CAD build for the part. Positions are in the model's coordinates, mm. Face numbers are marked on the shaded views. A direction names the side the tool comes from. Give positions to 0.01 mm unless a question says otherwise; leave off trailing zeros. Write each loop counter-clockwise with the first axis right and the second up, starting at its lowest first coordinate (ties: lowest second). Pieces come first, ordered by that corner, then holes. Notation, with made-up numbers: (69, 18) -> (112, 18) arc R20 ccw to (112, 42) -> close; hole circle Ø11 at (-1, 37.25). An arc over 180 degrees is marked (long way). Answer in a Markdown table with one row per item. Add a question column.
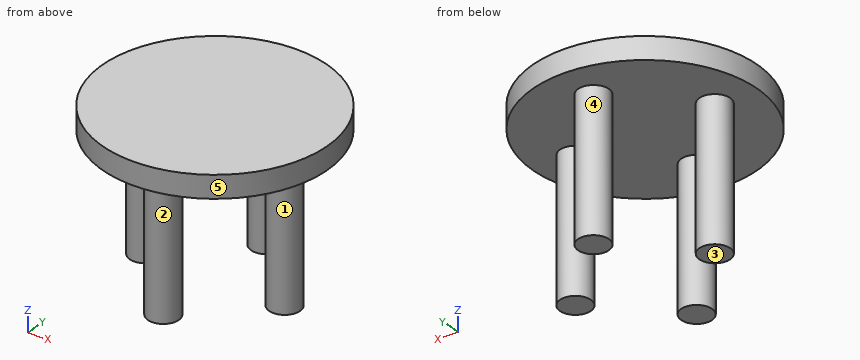
```python
from build123d import *

# Parameters (mm, degrees)
SKETCH_R     = 40
PAD_DEPTH    = 8
SKETCH001_R  = 5.5
PAD001_DEPTH = 50


with BuildPart() as part:
    # Sketch → Pad (new body)
    with BuildSketch(Plane.XY):
        Circle(SKETCH_R)
    extrude(amount=PAD_DEPTH)

    # Sketch001 → Pad001 (new body)
    with BuildSketch(Plane(origin=(0, 0, 0), x_dir=(1, 0, 0), z_dir=(0, 0, -1))):
        with Locations((0, 25)):
            Circle(SKETCH001_R)
        with Locations((-25, 0)):
            Circle(SKETCH001_R)
        with Locations((0, -25)):
            Circle(SKETCH001_R)
        with Locations((25, 0)):
            Circle(SKETCH001_R)
    extrude(amount=PAD001_DEPTH)


solid = part.part
```
Item 1: Drop flat-ended pins along their axis: pin 1 Ø8 at (y, z) = (22, -19) entering from +X; pin 2 Ø1 at (x, z) = (23, -39.5) entering from +Y; pin 3 Ø12 at (y, z) = (-21.5, -8.5) entering from -X. Give the stop position or say it passes through.
Item 2: Slice it at D-D, the plane y = -32. List the corners of the cut face in (x, z).
Item 3: Which spindle directions (+Z, -Z, +X, -X, +Y, -Y) get a long thin tool onto all of the face, cutting with end or side? Do the marked faces 4 and 5. Say none if no direction does.
Item 4: Probe L1, parallel to Z at x = -17, y = 12.5; L2, parallel to Y at x = -2.5, z = -10; L3, parallel to Y at x = 4.5, z = -3.5. List the from-to ranges inside material, lowest first. Write a range as from..to.
Item 5: Mould opens along X. For the marked faces 1, 2 and 3 say: released by +X, released by -X, zero draft, split by the parting line, or undercut.
Item 6: Slice it at A-A, the plane x = 0. List the corners of the cut face in (y, z).
Item 7: Slice it at B-B, the plane z = -17. List the corners of the cut face in (x, y).
Answer key:
| question | item | result |
|---|---|---|
| 1 | pin 1 | stops at x = 5.5 |
| 1 | pin 2 | stops at y = 5.29 |
| 1 | pin 3 | stops at x = -5.5 |
| 2 | outline | (-24, 0) -> (24, 0) -> (24, 8) -> (-24, 8) -> close |
| 3 | face 4 | -Z |
| 3 | face 5 | +Z, -Z |
| 4 | L1 | z = 0..8 |
| 4 | L2 | y = -29.9..-20.1, 20.1..29.9 |
| 4 | L3 | y = -28.16..-21.84, 21.84..28.16 |
| 5 | face 1 | undercut |
| 5 | face 2 | split by the parting line |
| 5 | face 3 | zero draft |
| 6 | outline | (-40, 0) -> (-30.5, 0) -> (-30.5, -50) -> (-19.5, -50) -> (-19.5, 0) -> (19.5, 0) -> (19.5, -50) -> (30.5, -50) -> (30.5, 0) -> (40, 0) -> (40, 8) -> (-40, 8) -> close |
| 7 | outline | circle Ø11 at (-25, 0); circle Ø11 at (0, -25); circle Ø11 at (0, 25); circle Ø11 at (25, 0) |
